Answer from the drawing. Dimensions are ordinates in mm from the lowest x, y and z of the part. A direction names the side the tool comes from. Give positions to 0.01 mm unless a question says otherwise; leave off trailing zeros. Order: outer loops, then holes, each group sorted by start corner. A loop starts at its lowest first (then second) coordinate and runs counter-clockwise, first axis right, second up.
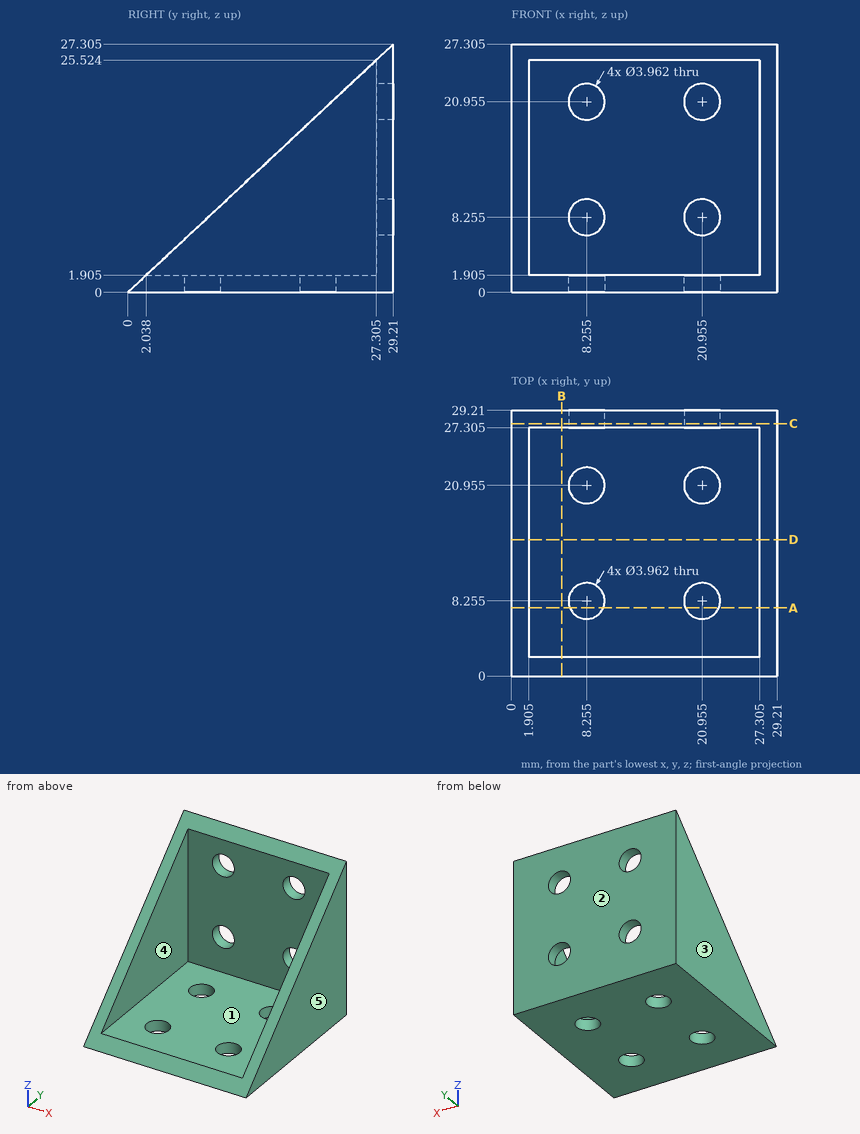
1. Given P1, Ø3, axis at x = 8.255, z = 8.255, coming from the +Y side; P2, Ø5, axis at x = 5, z = 18.5, coming from the -Y side (3 decimals); P3, Ø4.5, axis at x = 8.255, y = 20.955, coming from the +Z side (3 decimals); P4, Ø5, axis at x = 11, z = 3, coming from the -Y side (1 decimal), each flat-ended and moving along its own axis, determine where each tip first touches the part or whether it passes through.
Findings below:
P1: passes through
P2: stops at y = 27.305
P3: stops at z = 1.905
P4: stops at y = 0.5
2. The part is cut by section B-B (x = 5.5). Write down the section's boundary in (y, z) (1 decimal).
Findings below:
outline: (0, 0) - (29.2, 0) - (29.2, 27.3) - (27.3, 25.5) - (27.3, 1.9) - (2, 1.9) - close
3. The mould has two halves that part along X. Classify the marked faces 3, 4 and 5: pulls with the +X half, pulls with the -X half, needs draft (parallel to the pull), parting line crosses it, or undercut.
Findings below:
face 3: pulls with the -X half
face 4: undercut
face 5: pulls with the +X half
4. Straight lines are drawn through the part: probe 1 along X at (y, z) = (12.25, 3.75) (1 decimal); probe 2 along Y at (x, z) = (9.75, 10.75) (1 decimal); probe 3 along Z at (x, y) = (23, 7) (1 decimal). For each, find the intervals that lie inside material, in ascending order.
Findings below:
probe 1: x = 0 to 1.9, 27.3 to 29.2
probe 2: y = 27.3 to 29.2
probe 3: z = 0 to 1.9
5. Which of the six approach directions +Z, -Z, +X, -X, +Y, -Y give full straight-line access (tool end or side, diameter ignored) to the marked faces 1 and 2?
Findings below:
face 1: +Z, -Y
face 2: +Z, -Z, +X, -X, +Y
6. The part is cut by section D-D (y = 15). Write down the section's boundary in (x, z) (1 decimal).
Findings below:
outline: (0, 0) - (29.2, 0) - (29.2, 14) - (27.3, 14) - (27.3, 1.9) - (1.9, 1.9) - (1.9, 14) - (0, 14) - close
7. The part is cut by section C-C (y = 27.75). Write down the section's boundary in (x, z) (1 decimal).
Findings below:
outline: (0, 0) - (29.2, 0) - (29.2, 25.9) - (0, 25.9) - close; hole circle Ø4 at (8.3, 8.3); hole circle Ø4 at (8.3, 21); hole circle Ø4 at (21, 8.3); hole circle Ø4 at (21, 21)
8. The part is cut by section A-A (y = 7.5). Write down the section's boundary in (x, z) (1 decimal).
Findings below:
outline: (0, 0) - (6.4, 0) - (6.4, 1.9) - (1.9, 1.9) - (1.9, 7) - (0, 7) - close; (10.1, 0) - (19.1, 0) - (19.1, 1.9) - (10.1, 1.9) - close; (22.8, 0) - (29.2, 0) - (29.2, 7) - (27.3, 7) - (27.3, 1.9) - (22.8, 1.9) - close
